Design review of the part built by this model. Coordinates are the model's own, in mm. Coordinates: 2 decimals unless noted, no trailing zeros. Loops run counter-clockwise (first coordinate to the right, second up) from the corner with the lowest first, then second, coordinate; pieces in that order, holes last. Notation, with made-up numbers: (31.5, -36) -> (80.5, -36) arc R8 cw to (80.5, -32) -> close; hole circle Ø3 at (15.5, 47.25). An arc over 180 degrees is marked (long way). Answer as a JSON object with one key per item and string values.
```python
from build123d import *

# Parameters (mm, degrees)
SKETCH2_R                                  = 2
BOSS_EXTRUDE1_DEPTH                        = 5
CUT_EXTRUDE1_REACH                         = 73.718
SKETCH4_R                                  = 1
MIRROR2_COPY_1_REACH                       = 73.718
MIRROR2_COPY_1_SKETCH_R                    = 1
MIRROR2_AT_THE_SECOND_PLANE_COPY_1_REACH   = 73.718
MIRROR2_AT_THE_SECOND_PLANE_COPY_1_SKETC_R = 1
MIRROR2_AT_THE_SECOND_PLANE_COPY_2_REACH   = 73.718
MIRROR2_AT_THE_SECOND_PLANE_COPY_2_SKETC_R = 1
MIRROR2_AT_THE_SECOND_PLANE_COPY_3_REACH   = 73.718
MIRROR2_AT_THE_SECOND_PLANE_COPY_3_SKETC_R = 1


with BuildPart() as part:
    # Sketch2 → Boss-Extrude1 (new body)
    # profile 1 of 2: a face of its own
    with BuildSketch(Plane(origin=(0, 0, 0), x_dir=(1, 0, 0), z_dir=(0, 1, 0))):
        with BuildLine():
            ThreePointArc((37.5, -45.5), (36.085786438, -42.085786438), (39.5, -43.5))
            Line((39.5, -43.5), (47.5, -43.5))
            Line((47.5, -43.5), (47.5, 53.5))
            Line((47.5, 53.5), (-47.5, 53.5))
            Line((-47.5, 53.5), (-47.5, -53.5))
            Line((-47.5, -53.5), (37.5, -53.5))
            Line((37.5, -53.5), (37.5, -45.5))
        make_face()
        with Locations(Location((-37.5, -43.5, 0), (0, 0, 270))):
            Circle(SKETCH2_R, mode=Mode.SUBTRACT)
        with Locations(Location((-37.5, 43.5, 0), (0, 0, 270))):
            Circle(SKETCH2_R, mode=Mode.SUBTRACT)
        with Locations(Location((37.5, 43.5, 0), (0, 0, 270))):
            Circle(SKETCH2_R, mode=Mode.SUBTRACT)
    # profile 2 of 2: a face of its own
    with BuildSketch(Plane(origin=(0, 0, 0), x_dir=(1, 0, 0), z_dir=(0, 1, 0))):
        with BuildLine():
            Line((47.5, -43.5), (39.5, -43.5))
            ThreePointArc((39.5, -43.5), (38.914213562, -44.914213562), (37.5, -45.5))
            Line((37.5, -45.5), (37.5, -53.5))
            Line((37.5, -53.5), (47.5, -53.5))
            Line((47.5, -53.5), (47.5, -43.5))
        make_face()
    extrude(amount=BOSS_EXTRUDE1_DEPTH)

    # Sketch4 → Cut-Extrude1 (cut, up to next)
    with BuildSketch(Plane(origin=(0, 5, 0), x_dir=(1, 0, 0), z_dir=(0, 1, 0)), mode=Mode.PRIVATE) as cut_extrude1_sk1:
        with Locations(Location((42.63, 46.04, 0), (0, 0, 270))):
            Circle(SKETCH4_R)
    cut_extrude1_tool1 = extrude(cut_extrude1_sk1.sketch, amount=-CUT_EXTRUDE1_REACH, mode=Mode.PRIVATE) & part.part
    cut_extrude1 = cut_extrude1_tool1.solids().sort_by_distance((42.63, 5, -46.04))[0]
    add(cut_extrude1, mode=Mode.SUBTRACT)

    # Mirror1: Cut-Extrude1 across plane
    add(cut_extrude1.mirror(Plane(origin=(0, 0, -28.738611276), x_dir=(1, 0, 0), z_dir=(0, 0, -1))), mode=Mode.SUBTRACT)

    # Mirror2: Cut-Extrude1 across plane
    add(cut_extrude1.mirror(Plane(origin=(0, 0, 0), x_dir=(0, 0, 1), z_dir=(1, 0, 0))), mode=Mode.SUBTRACT)

    # Mirror2 copy 1 sketch → Mirror2 copy 1 (cut, up to next)
    with BuildSketch(Plane(origin=(0, 5, -57.477222552), x_dir=(-1, 0, 0), z_dir=(0, 1, 0)), mode=Mode.PRIVATE) as mirror2_copy_1_sk1:
        with Locations(Location((42.63, 46.04, 0), (0, 0, 270))):
            Circle(MIRROR2_COPY_1_SKETCH_R)
    mirror2_copy_1_tool1 = extrude(mirror2_copy_1_sk1.sketch, amount=-MIRROR2_COPY_1_REACH, mode=Mode.PRIVATE) & part.part
    add(mirror2_copy_1_tool1.solids().sort_by_distance((-42.63, 5, -11.437222552))[0], mode=Mode.SUBTRACT)

    # Mirror2 at the second plane: Cut-Extrude1 across plane
    add(cut_extrude1.mirror(Plane.XY), mode=Mode.SUBTRACT)

    # Mirror2 at the second plane copy 1 sketc → Mirror2 at the second plane copy 1 (cut, up to next)
    with BuildSketch(Plane(origin=(0, 5, 57.477222552), x_dir=(1, 0, 0), z_dir=(0, 1, 0)), mode=Mode.PRIVATE) as mirror2_at_the_second_plane_copy_1_sk1:
        with Locations(Location((42.63, 46.04, 0), (0, 0, 270))):
            Circle(MIRROR2_AT_THE_SECOND_PLANE_COPY_1_SKETC_R)
    mirror2_at_the_second_plane_copy_1_tool1 = extrude(mirror2_at_the_second_plane_copy_1_sk1.sketch, amount=-MIRROR2_AT_THE_SECOND_PLANE_COPY_1_REACH, mode=Mode.PRIVATE) & part.part
    add(mirror2_at_the_second_plane_copy_1_tool1.solids().sort_by_distance((42.63, 5, 11.437222552))[0], mode=Mode.SUBTRACT)

    # Mirror2 at the second plane copy 2 sketc → Mirror2 at the second plane copy 2 (cut, up to next)
    with BuildSketch(Plane(origin=(0, 5, 0), x_dir=(-1, 0, 0), z_dir=(0, 1, 0)), mode=Mode.PRIVATE) as mirror2_at_the_second_plane_copy_2_sk1:
        with Locations(Location((42.63, 46.04, 0), (0, 0, 270))):
            Circle(MIRROR2_AT_THE_SECOND_PLANE_COPY_2_SKETC_R)
    mirror2_at_the_second_plane_copy_2_tool1 = extrude(mirror2_at_the_second_plane_copy_2_sk1.sketch, amount=-MIRROR2_AT_THE_SECOND_PLANE_COPY_2_REACH, mode=Mode.PRIVATE) & part.part
    add(mirror2_at_the_second_plane_copy_2_tool1.solids().sort_by_distance((-42.63, 5, 46.04))[0], mode=Mode.SUBTRACT)

    # Mirror2 at the second plane copy 3 sketc → Mirror2 at the second plane copy 3 (cut, up to next)
    with BuildSketch(Plane(origin=(0, 5, 57.477222552), x_dir=(-1, 0, 0), z_dir=(0, 1, 0)), mode=Mode.PRIVATE) as mirror2_at_the_second_plane_copy_3_sk1:
        with Locations((42.63, -46.04)):
            Circle(MIRROR2_AT_THE_SECOND_PLANE_COPY_3_SKETC_R)
    mirror2_at_the_second_plane_copy_3_tool1 = extrude(mirror2_at_the_second_plane_copy_3_sk1.sketch, amount=-MIRROR2_AT_THE_SECOND_PLANE_COPY_3_REACH, mode=Mode.PRIVATE) & part.part
    add(mirror2_at_the_second_plane_copy_3_tool1.solids().sort_by_distance((-42.63, 5, 11.437222552))[0], mode=Mode.SUBTRACT)


solid = part.part
```
1) Wall thickness on probe 1 along Z at (x, y) = (-42.63, 3.4); probe 2 along X at (y, z) = (2.85, -43.5); probe 3 along Z at (x, y) = (37, 0.7): over which ranges is each line inside the solid? List them lowest first.
Completed:
{"probe 1": "-53.5 to -47.04, -45.04 to -12.44, -10.44 to 10.44, 12.44 to 45.04, 47.04 to 53.5", "probe 2": "-47.5 to -39.5, -35.5 to 35.5, 39.5 to 47.5", "probe 3": "-53.5 to -45.44, -41.56 to 41.56, 45.44 to 53.5"}
2) The part is to be moulded in two halves that separate along X. For faces 1 (the cylindrical face through (-39.452, 2.465, -43.934)), 2 (the flat face through (-47.5, 2, -1)), 3 (the flat face through (-1, 2, 53.5)), 4 (the flat face through (47.5, 2, 1)), say which applies: pulls with the +X half, pulls with the -X half, needs draft (parallel to the pull), parting line crosses it, or undercut.
Completed:
{"face 1": "undercut", "face 2": "pulls with the -X half", "face 3": "needs draft", "face 4": "pulls with the +X half"}
3) Add section A-A, the plane z = -43.5. Give the boundary of the cut face in (x, y), and give its area (3 significant figures).
Completed:
{"outline": "(-47.5, 0) -> (-39.5, 0) -> (-39.5, 5) -> (-47.5, 5) -> close; (-35.5, 0) -> (35.5, 0) -> (35.5, 5) -> (-35.5, 5) -> close; (39.5, 0) -> (47.5, 0) -> (47.5, 5) -> (39.5, 5) -> close", "area": "435 mm²"}
4) Clearance check with a flat-ended pin moving along its axis: pin 1 Ø1.6 at (x, z) = (-42.63, 46.04) entering from +Y. State where the tip first meets the part, or that it passes through.
Completed:
{"pin 1": "through"}
5) Add section B-B, the plane x = -37.5. Give the boundary of the cut face in (y, z).
Completed:
{"outline": "(0, -53.5) -> (5, -53.5) -> (5, -45.5) -> (0, -45.5) -> close; (0, -41.5) -> (5, -41.5) -> (5, 41.5) -> (0, 41.5) -> close; (0, 45.5) -> (5, 45.5) -> (5, 53.5) -> (0, 53.5) -> close"}
